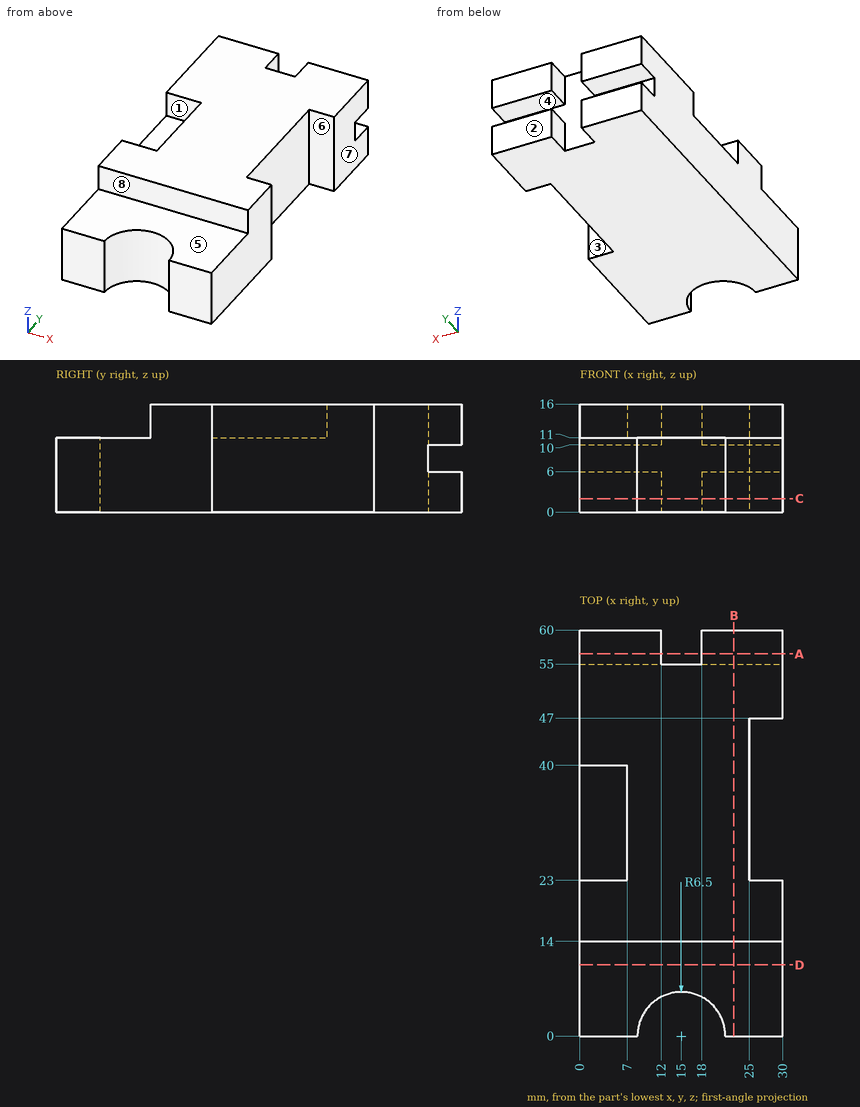
Input: dimensioned drawing with shaded views. Units: mm. Origin: part minimum x, y, z. A direction names the side the tool comes from. Coordinates: 2 decimals unless noted, no trailing zeros. Loops run counter-clockwise (first coordinate to the right, second up) from the corner with the lowest first, then second, coordinate; pieces in that order, holes last. Notation, with made-up numbers: M 45.5,73.5 L 57.5,73.5 A27 ccw 57.5,107.5 Z; hole C 70,4 d8. An arc over 180 degrees is marked long. Use a Markdown table: item, result. Add a question column.
Q1. First-contact query: pin 1 (5.5 mm diameter, centred on x = 28, z = 10, fed in from -Y); pin 2 (1.5 mm diameter, centred on x = 15.5, z = 11, fed in from -Y); pin 3 (2 mm diameter, centred on x = 4.5, y = 35, fed in from +Z); pin 4 (6 mm diameter, centred on x = 14, z = 9.5, fed in from -Y). Flat tips, straight axial feed; report the tip coordinate or a pass-through.
Q2. Draft query along Y for the marked faces 6, 7 and 8. Return one class per face: pulls with the +Y half, pulls with the -Y half, needs draft (parallel to the pull), parting line crosses it, or undercut.
Q3. Material intervals for L1, parallel to Z at x = 8.5, y = 55.5; L2, parallel to Y at x = 1.75, z = 7.75; L3, parallel to X at y = 25.5, z = 14, sorted ascending.
Q4. Section query A-A, the plane y = 56.5. Return loops of the section in (x, z).
Q5. Access query for the marked faces 1, 2, 3, 4 and 5. Directions: +Z, -Z, +X, -X, +Y, -Y. A direction counts if a zero-diameter tool reaches every point of the face in a straight line with its end or side. Return the directions, or none.
Q6. Section query D-D, the plane y = 10.5. Return loops of the section in (x, z), and give its area (3 significant figures).
Q7. Section query B-B, the plane x = 22.75. Return loops of the section in (y, z), and give its area (3 significant figures).
Q8. Section query C-C, the plane z = 2. Return loops of the section in (x, y).
Result:
| question | item | result |
|---|---|---|
| 1 | pin 1 | stops at y = 0 |
| 1 | pin 2 | stops at y = 6.38 |
| 1 | pin 3 | stops at z = 11 |
| 1 | pin 4 | stops at y = 5.12 |
| 2 | face 6 | undercut |
| 2 | face 7 | needs draft |
| 2 | face 8 | pulls with the -Y half |
| 3 | L1 | z = 0 to 6, 10 to 16 |
| 3 | L2 | y = 0 to 55 |
| 3 | L3 | x = 7 to 25 |
| 4 | outline | M 0,0 L 12,0 L 12,6 L 0,6 Z; M 0,10 L 12,10 L 12,16 L 0,16 Z; M 18,0 L 30,0 L 30,6 L 18,6 Z; M 18,10 L 30,10 L 30,16 L 18,16 Z |
| 5 | face 1 | +Z, -X |
| 5 | face 2 | +Z, -Z, +X, -X, +Y |
| 5 | face 3 | +Z, -Z, +X |
| 5 | face 4 | +X, -X, +Y |
| 5 | face 5 | +Z, +X, -X, -Y |
| 6 | outline | M 0,0 L 30,0 L 30,11 L 0,11 Z |
| 6 | area | 330 mm2 |
| 7 | outline | M 0,0 L 60,0 L 60,6 L 55,6 L 55,10 L 60,10 L 60,16 L 14,16 L 14,11 L 0,11 Z |
| 7 | area | 870 mm2 |
| 8 | outline | M 0,0 L 8.5,0 A6.5 cw 21.5,0 L 30,0 L 30,23 L 25,23 L 25,47 L 30,47 L 30,60 L 18,60 L 18,55 L 12,55 L 12,60 L 0,60 Z |
